Here's the drawing with two shaded views (mm, measured from the low corner). I have some questions. A direction names the side the tool comes from. Give positions to 0.01 mm unless a question says otherwise; leave off trailing zeros. Loops run counter-clockwise (first coordinate to the right, second up) from the corner with the lowest first, then second, coordinate; pieces in that order, holes last. Notation, with made-up numbers: (61.25, 31) - (85.25, 31) arc R22 cw to (85.25, 48) - close; hole circle Ø7 at (41.5, -17.5). An arc over 180 degrees is marked (long way). Use a Markdown table: item, result. Add a question column.
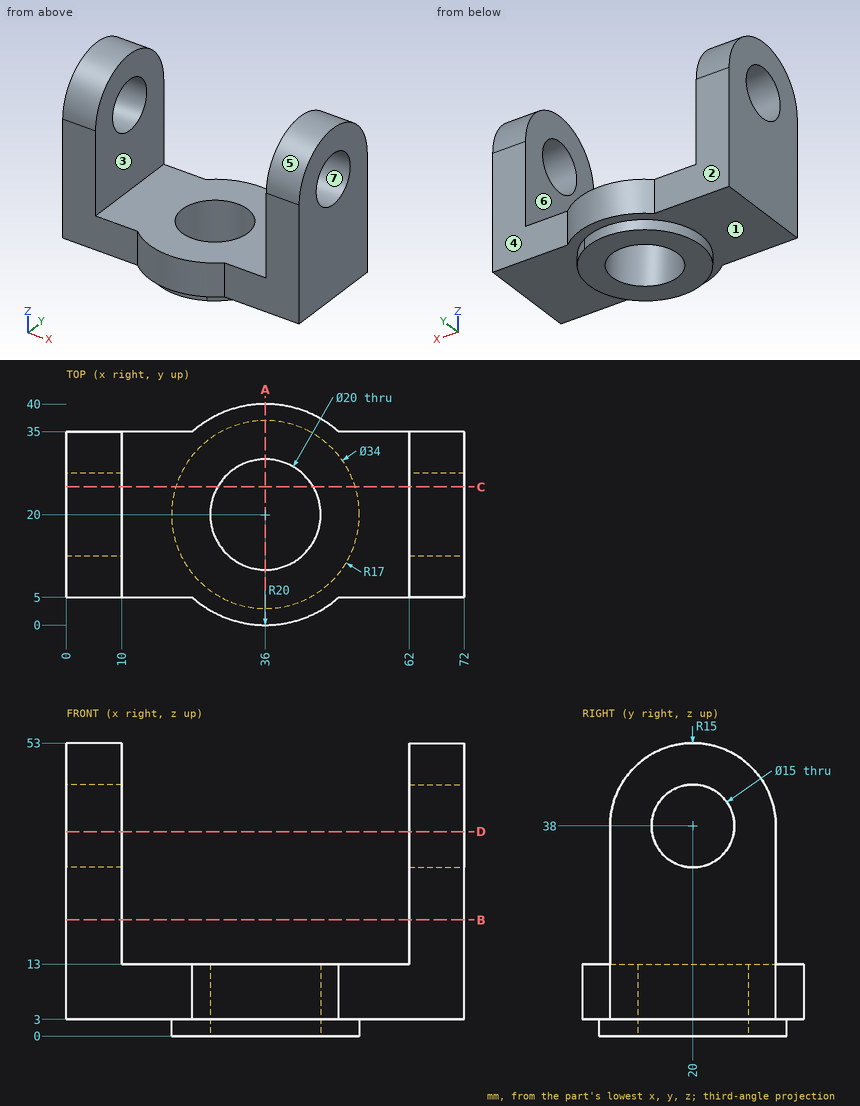
1. Suppose I cut it at B-B (z = 21). List the corners of the cut face in (x, y) for me.
2. Suppose I cut it at D-D (z = 37). List the corners of the cut face in (x, y) for me.
3. If we mould it in two halves opening along Z, with no side actions, what happens to the marked faces 5, 6 and 7? For each: released by +Z, released by -Z, zero draft, split by the parting line, or undercut.
4. Please list where these lines run through material, in increasing order: line 1 along X through (y, z) = (27.5, 29.5); line 2 along Z through (x, y) = (4, 20); line 3 along Z through (x, y) = (22, 10). Write a range as [from, to].
5. Suppose I cut it at C-C (y = 25). List the corners of the cut face in (x, z) for me.
6. Suppose I cut it at A-A (x = 36). List the corners of the cut face in (y, z) for me, and give its area (3 significant figures).
7. Will these pins go through, and if not, where does the flat tip stop? P1, Ø11.5, axis at x = 13, z = 23.5, coming from the +Y side; P2, Ø10, axis at x = 51, z = 6, coming from the -Y side; P3, Ø5, axis at x = 20.5, y = 36, coming from the -Z side.
8. On a 3-axis mill with a long thin cutter (end or side, diameter ignored), from which of +Z, -Z, +X, -X, +Y, -Y can I reach the whole of each face in a straight line? I mean the marked faces 1, 2, 3 and 4. Say none if no direction works.
Results below:
| question | item | result |
|---|---|---|
| 1 | outline | (0, 5) - (10, 5) - (10, 35) - (0, 35) - close; (62, 5) - (72, 5) - (72, 35) - (62, 35) - close |
| 2 | outline | (0, 5) - (10, 5) - (10, 12.57) - (0, 12.57) - close; (0, 27.43) - (10, 27.43) - (10, 35) - (0, 35) - close; (62, 5) - (72, 5) - (72, 12.57) - (62, 12.57) - close; (62, 27.43) - (72, 27.43) - (72, 35) - (62, 35) - close |
| 3 | face 5 | released by +Z |
| 3 | face 6 | zero draft |
| 3 | face 7 | undercut |
| 4 | line 1 | [0, 10], [62, 72] |
| 4 | line 2 | [3, 30.5], [45.5, 53] |
| 4 | line 3 | [3, 13] |
| 5 | outline | (0, 3) - (19.75, 3) - (19.75, 0) - (27.34, 0) - (27.34, 13) - (10, 13) - (10, 32.41) - (0, 32.41) - close; (0, 43.59) - (10, 43.59) - (10, 52.14) - (0, 52.14) - close; (44.66, 0) - (52.25, 0) - (52.25, 3) - (72, 3) - (72, 32.41) - (62, 32.41) - (62, 13) - (44.66, 13) - close; (62, 43.59) - (72, 43.59) - (72, 52.14) - (62, 52.14) - close |
| 6 | outline | (0, 3) - (3, 3) - (3, 0) - (10, 0) - (10, 13) - (0, 13) - close; (30, 0) - (37, 0) - (37, 3) - (40, 3) - (40, 13) - (30, 13) - close |
| 6 | area | 242 mm² |
| 7 | P1 | y = 35 |
| 7 | P2 | y = 2.68 |
| 7 | P3 | z = 3 |
| 8 | face 1 | -Z |
| 8 | face 2 | +Z, -Z, -X, +Y |
| 8 | face 3 | +Z, +Y, -Y |
| 8 | face 4 | +Z, -Z, +X, +Y |
